Part model, mm, in its own coordinate system. A direction names the side the tool comes from. Round coordinates to 2 decimals unless told otherwise and drop trailing zeros. Write each loop counter-clockwise with the first axis right and the second up, starting at its lowest first coordinate (ties: lowest second). Pieces come first, ordered by that corner, then holes. Notation, with made-up numbers: M -18.5,39.5 L 38.5,39.5 A22 ccw 38.5,67.5 Z; hole C 89,8.25 d8. An arc over 180 degrees is marked long. One line per question, with ' | ' between items. Start each with the question number.
1) Drop a flat-ended pin along its axis: pin 1 Ø3 at (x, y) = (50, -179.32) entering from +Z. Give the stop position or say it passes through.
2) Mould opens along Y. For faces 1 (the face through (-111.1, -85.19, 0.74)), 2 (the face through (-138, 45, 0)) say: pulls with the +Y half, pulls with the -Y half, needs draft (parallel to the pull), parting line crosses it, or undercut.
3) Saw through at A-A (y = 0). List the corners of the cut face in (x, z), plus the area to 3 significant figures.
4) Wall check: probe 1 along Y at (x, z) = (100, 1.15); probe 2 along Y at (x, z) = (0, 0.95); probe 3 along X at (y, z) = (-148, 0.4). Give the ranges that are in metal, low to high. Write a range as [from, to].
5) Saw through at B-B (x = 112). List the corners of the cut face in (y, z), plus the area to 3 significant figures.
6) Saw through at C-C (z = 0.85). Give the number of separate pieces and of enclosed holes in the cut face, plus the area to 3 significant figures.
7) Tool access for faces 3 (the face through (-138, 45, 1.5)), 4 (the face through (-224.614, 164.055, 0.74)): list every direction of +Z, -Z, +X, -X, +Y, -Y with a clear straight run to the whole face (end or side of a thin tool).
```python
from build123d import *

# Parameters (mm, degrees)
F0_R     = 2
F0_R_2   = 3.15
F0_R_3   = 140
F1_DEPTH = 1.5


with BuildPart() as f1:
    # F0 (on Top) → F1 (new body)
    with BuildSketch(Plane.XY):
        with BuildLine():
            Line((-160.457017, -148.356514), (-287, -179.32))
            Line((-287, -179.32), (-277, -189.32))
            Line((-277, -189.32), (277, -189.32))
            Line((277, -189.32), (287, -179.32))
            Line((287, -179.32), (160.457017, -148.356514))
            ThreePointArc((160.457017, -148.356514), (157.517789, -147.769673), (160.496498, -148.102445))
            Line((160.496498, -148.102445), (290.47, -157))
            Line((290.47, -157), (300.47, -147))
            Line((300.47, -147), (300.47, 147))
            Line((300.47, 147), (290.47, 157))
            Line((290.47, 157), (160.496498, 148.102445))
            ThreePointArc((160.496498, 148.102445), (157.517789, 147.769673), (160.457017, 148.356514))
            Line((160.457017, 148.356514), (287, 179.32))
            Line((287, 179.32), (277, 189.32))
            Line((277, 189.32), (-277, 189.32))
            Line((-277, 189.32), (-287, 179.32))
            Line((-287, 179.32), (-160.457017, 148.356514))
            ThreePointArc((-160.457017, 148.356514), (-157.517789, 147.769673), (-160.496498, 148.102445))
            Line((-160.496498, 148.102445), (-290.47, 157))
            Line((-290.47, 157), (-300.47, 147))
            Line((-300.47, 147), (-300.47, -147))
            Line((-300.47, -147), (-290.47, -157))
            Line((-290.47, -157), (-160.496498, -148.102445))
            ThreePointArc((-160.496498, -148.102445), (-157.517789, -147.769673), (-160.457017, -148.356514))
        make_face()
        with Locations((-150, -179.32)):
            Circle(F0_R, mode=Mode.SUBTRACT)
        with Locations((-100, -179.32)):
            Circle(F0_R, mode=Mode.SUBTRACT)
        with Locations((-50, -179.32)):
            Circle(F0_R, mode=Mode.SUBTRACT)
        with Locations((-134.5, -77.5)):
            Circle(F0_R_2, mode=Mode.SUBTRACT)
        with Locations((0, -179.32)):
            Circle(F0_R, mode=Mode.SUBTRACT)
        with Locations((50, -179.32)):
            Circle(F0_R, mode=Mode.SUBTRACT)
        with Locations((100, -179.32)):
            Circle(F0_R, mode=Mode.SUBTRACT)
        with Locations((150, -179.32)):
            Circle(F0_R, mode=Mode.SUBTRACT)
        with Locations((134.5, -77.5)):
            Circle(F0_R_2, mode=Mode.SUBTRACT)
        with Locations((-134.5, 77.5)):
            Circle(F0_R_2, mode=Mode.SUBTRACT)
        Circle(F0_R_3, mode=Mode.SUBTRACT)
        with Locations((134.5, 77.5)):
            Circle(F0_R_2, mode=Mode.SUBTRACT)
    extrude(amount=F1_DEPTH)


solid = f1.part
```
Answer key:
1) pin 1: passes through
2) face 1: undercut | face 2: needs draft
3) outline: M -300.47,0 L -140,0 L -140,1.5 L -300.47,1.5 Z; M 140,0 L 300.47,0 L 300.47,1.5 L 140,1.5 Z | area: 481 mm2
4) probe 1: y = [-189.32, -181.32], [-177.32, -97.98], [97.98, 189.32] | probe 2: y = [-189.32, -181.32], [-177.32, -140], [140, 189.32] | probe 3: x = [-299.47, -160.5], [-157.5, 157.5], [160.5, 299.47]
5) outline: M -189.32,0 L -84,0 L -84,1.5 L -189.32,1.5 Z; M 84,0 L 189.32,0 L 189.32,1.5 L 84,1.5 Z | area: 316 mm2
6) separate pieces: 1 | enclosed holes: 12 | area: 158,000 mm2
7) face 3: +Z, +X, -X, +Y, -Y | face 4: +Z, -Z
